Check sheet for the modelled part. Datum: model origin and axes. Units: mm. Face numbers are marked on the shaded views. A direction names the side the tool comes from. Give positions to 0.01 mm unless a question says otherwise; leave off trailing zeros. Order: outer loops, then holes, each group sorted by start corner. A loop starts at its lowest first (then second) coordinate and runs counter-clockwise, first axis right, second up.
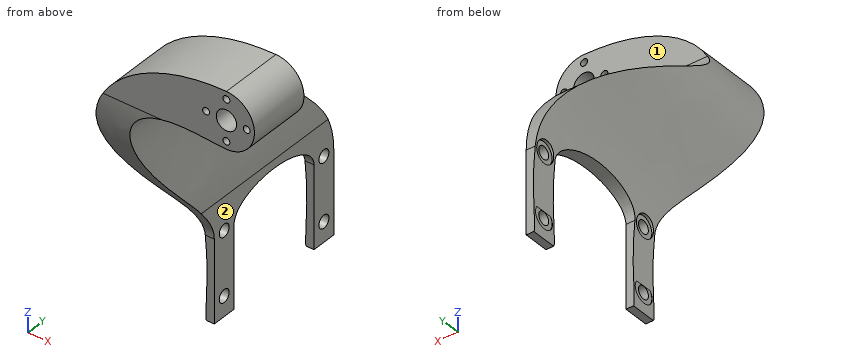
from build123d import *

# Parameters (mm, degrees)
BOSS_EXTRUDE1_START = -78.5
BOSS_EXTRUDE1_DEPTH = 157
SKETCH5_W           = 473.004377806
SKETCH5_H           = 558.860634618
CUT_EXTRUDE1_DEPTH  = 109.5
SKETCH6_R           = 1.36
SKETCH6_R_2         = 4
CUT_EXTRUDE2_DEPTH  = 25
SKETCH7_R           = 2.5
CUT_EXTRUDE3_DEPTH  = 10
SKETCH8_R           = 4.25
CUT_EXTRUDE4_DEPTH  = 2


# Read off the part's stored shape, not the designer's step: Boss-Extrude1
with BuildPart() as part:
    # Boss-Extrude1 outline → Boss-Extrude1 (new body)
    with BuildSketch(Plane.XZ.offset(BOSS_EXTRUDE1_START)):
        with BuildLine():
            ThreePointArc((0, -11.05), (11.05, 0), (0, 11.05))
            add(Edge.make_bspline(
                [(0, 11.05), (-73.705988569, 11.05), (-70.075162013, -66.476999877), (-19.953361107, -14.552256493), (-38.925778701, -112.613618432), (-35.925778701, -112.613618432)],
                knots=[0, 0, 0, 0, 0, 0, 1, 1, 1, 1, 1, 1], degree=5))
            Line((-35.925778701, -112.613618432), (-32.925778701, -112.613618432))
            Line((-32.925778701, -112.613618432), (-32.925778701, -66.813618432))
            add(Edge.make_bspline(
                [(-32.925778701, -66.813618432), (-32.925778701, -47.05), (-63.009039822, 1.033261121), (-14.925778701, -11.05), (0, -11.05)],
                knots=[0, 0, 0, 0, 0, 1, 1, 1, 1, 1], degree=4))
        make_face()
    extrude(amount=BOSS_EXTRUDE1_DEPTH)

    # Sketch5 → Cut-Extrude1 (cut, symmetric)
    with BuildSketch(Plane.ZY):
        with Locations((-57.495001252, 3.891745074)):
            Rectangle(SKETCH5_W, SKETCH5_H)
        with BuildLine():
            Line((-117.55, 11.0465), (-80.216666667, 11.0465))
            add(Edge.make_bspline(
                [(-11.05, -25), (-46.05, -25), (-65.216666667, 11.0465), (-80.216666667, 11.0465)],
                knots=[0, 0, 0, 0, 1, 1, 1, 1], degree=3))
            Line((-11.05, -25), (11.05, -25))
            Line((11.05, -25), (11.05, 0))
            Line((11.05, 0), (-11.05, 0))
            add(Edge.make_bspline(
                [(-11.05, 0), (-26.05, 0), (-40.216666667, 71.3715), (-80.216666667, 71.3715)],
                knots=[0, 0, 0, 0, 1, 1, 1, 1], degree=3))
            Line((-80.216666667, 71.3715), (-117.55, 71.3715))
            Line((-117.55, 71.3715), (-117.55, 61.3715))
            Line((-117.55, 61.3715), (-80.216666667, 61.3715))
            add(Edge.make_bspline(
                [(-80.216666667, 21.0465), (-70.133333333, 21.0465), (-70.133333333, 41.209), (-70.133333333, 61.3715), (-80.216666667, 61.3715)],
                knots=[3.141592654, 3.141592654, 3.141592654, 4.71238898, 4.71238898, 6.283185307, 6.283185307, 6.283185307], degree=2, weights=[1, 0.707106781, 1, 0.707106781, 1]))
            Line((-80.216666667, 21.0465), (-117.55, 21.0465))
            Line((-117.55, 21.0465), (-117.55, 11.0465))
        make_face(mode=Mode.SUBTRACT)
    extrude(amount=CUT_EXTRUDE1_DEPTH, both=True, mode=Mode.SUBTRACT)

    # Sketch6 → Cut-Extrude2 (cut)
    with BuildSketch(Plane.XZ.offset(25)):
        with Locations(Location((0, 8, 0), (0, 0, 270))):
            Circle(SKETCH6_R)
        with Locations(Location((0, 0, 0), (0, 0, 270))):
            Circle(SKETCH6_R_2)
        with Locations(Location((8, 0, 0), (0, 0, 270))):
            Circle(SKETCH6_R)
        with Locations(Location((-8, 0, 0), (0, 0, 270))):
            Circle(SKETCH6_R)
        with Locations(Location((0, -8, 0), (0, 0, 270))):
            Circle(SKETCH6_R)
    extrude(amount=-CUT_EXTRUDE2_DEPTH, mode=Mode.SUBTRACT)

    # Sketch7 → Cut-Extrude3 (cut)
    with BuildSketch(Plane(origin=(-32.925778701, 0, 0), x_dir=(0, 0, -1), z_dir=(1, 0, 0))):
        with Locations((79.713618432, 66.3715)):
            Circle(SKETCH7_R)
        with Locations((104.713618432, 66.3715)):
            Circle(SKETCH7_R)
        with Locations((104.713618432, 16.0465)):
            Circle(SKETCH7_R)
        with Locations((79.713618432, 16.0465)):
            Circle(SKETCH7_R)
    extrude(amount=-CUT_EXTRUDE3_DEPTH, mode=Mode.SUBTRACT)

    # Sketch8 → Cut-Extrude4 (cut)
    with BuildSketch(Plane(origin=(-37.925778701, 0, 0), x_dir=(0, 0, -1), z_dir=(1, 0, 0))):
        with Locations(Location((79.713618432, 66.3715, 0), (0, 0, 180))):
            Circle(SKETCH8_R)
        with Locations((104.713618432, 66.3715)):
            Circle(SKETCH8_R)
        with Locations((104.713618432, 16.0465)):
            Circle(SKETCH8_R)
        with Locations(Location((79.713618432, 16.0465, 0), (0, 0, 180))):
            Circle(SKETCH8_R)
    extrude(amount=CUT_EXTRUDE4_DEPTH, mode=Mode.SUBTRACT)


solid = part.part
1) Set-up check for the marked faces 1 and 2: record each of +Z, -Z, +X, -X, +Y, -Y from which the full face is reachable in a straight line by a thin tool's end or side.
Recorded:
face 1: +Z, +X, -X, +Y
face 2: +Z, -Z, +X, +Y, -Y
2) Depth check by flat-ended pin: pin 1 Ø5.5 at (y, z) = (17.5, -105.5) entering from -X; pin 2 Ø4.5 at (x, z) = (-8, 0) entering from +Y; pin 3 Ø1.1 at (x, z) = (-34, -102) entering from -Y. Enter the tip coordinate at first touch or a pass-through.
Recorded:
pin 1: stops at x = -36.16
pin 2: stops at y = 0
pin 3: stops at y = 11.05
3) Section check B-B, the plane y = -14.5. State how many separate pieces and enclosed holes the cut face has, then the cut area to 3 significant figures.
Recorded:
separate pieces: 1
enclosed holes: 5
area: 1,310 mm2
4) Section check A-A, the plane x = 8. Record the cut outline in (y, z), then the cut area to 3 significant figures.
Recorded:
outline: (-25, -7.62) - (0, -7.62) - (0, -1.36) - (-25, -1.36) - close; (-25, 1.36) - (0, 1.36) - (0, 7.62) - (-25, 7.62) - close
area: 313 mm2
5) Material ranges on L1, parallel to Y at x = -27, z = 4.5; L2, parallel to Z at x = -44, y = -10; L3, parallel to X at y = 64, z = -100.5, recorded low to high.
Recorded:
L1: y = -25 to 0
L2: z = -49.32 to -4.91
L3: x = -35.87 to -32.93
